```python
from build123d import *

# Parameters (mm, degrees)
BOSS_EXTRUDE1_DEPTH = 2
SKETCH2_R           = 2
CUT_EXTRUDE1_DEPTH  = 3
SKETCH6_W           = 5
SKETCH6_H           = 30
BOSS_EXTRUDE2_DEPTH = 10
FILLET1_R           = 5
FILLET2_R           = 3


with BuildPart() as part:
    # Sketch1 → Boss-Extrude1 (new body)
    with BuildSketch(Plane.XY):
        with BuildLine():
            Line((-43, 260), (43, 260))
            ThreePointArc((43, 260), (50.071067812, 262.928932188), (53, 270))
            Line((53, 270), (53, 350))
            ThreePointArc((53, 350), (50.071067812, 357.071067812), (43, 360))
            Line((43, 360), (-43, 360))
            ThreePointArc((-43, 360), (-50.071067812, 357.071067812), (-53, 350))
            Line((-53, 350), (-53, 270))
            ThreePointArc((-53, 270), (-50.071067812, 262.928932188), (-43, 260))
        make_face()
    extrude(amount=-BOSS_EXTRUDE1_DEPTH)

    # Sketch2 → Cut-Extrude1 (cut)
    with BuildSketch(Plane(origin=(0, 0, -2), x_dir=(-1, 0, 0), z_dir=(0, 0, -1))):
        with Locations((46, 267)):
            Circle(SKETCH2_R)
        with Locations((-46, 267)):
            Circle(SKETCH2_R)
        with Locations(Location((-46, 353, 0), (0, 0, 180))):
            Circle(SKETCH2_R)
        with Locations(Location((46, 353, 0), (0, 0, 180))):
            Circle(SKETCH2_R)
    extrude(amount=-CUT_EXTRUDE1_DEPTH, mode=Mode.SUBTRACT)

    # Sketch6 → Boss-Extrude2 (add)
    with BuildSketch(Plane.XY):
        with Locations((0, 310)):
            Rectangle(SKETCH6_W, SKETCH6_H)
    extrude(amount=BOSS_EXTRUDE2_DEPTH)

    # Fillet1
    fillet1_edges = [part.edges().sort_by_distance(p)[0] for p in [
        (0, 295, 10),
        (0, 325, 10),
    ]]
    fillet(fillet1_edges, radius=FILLET1_R)

    # Fillet2
    fillet2_edges = [part.edges().sort_by_distance(p)[0] for p in [
        (0, 295, 0),
        (0, 325, 0),
    ]]
    fillet(fillet2_edges, radius=FILLET2_R)


solid = part.part
```
For this review, take the finished solid that the model builds, in its own axes (mm). A direction names the side the tool comes from. Round coordinates to 2 decimals unless told otherwise and drop trailing zeros. Write each loop counter-clockwise with the first axis right and the second up, starting at its lowest first coordinate (ties: lowest second). Pieces come first, ordered by that corner, then holes. Notation, with made-up numbers: M 68.5,14 L 84.5,14 A21 cw 84.5,42 Z; hole C 3.5,30.25 d7. An arc over 180 degrees is marked long. One line per item, written item: value. Start each with the question number.
(1) Insertion check: pin 1 (3 mm diameter, centred on y = 283.5, z = 0.5, fed in from +X); pin 2 (5 mm diameter, centred on x = 46, y = 267, fed in from +Z); pin 3 (0.6 mm diameter, centred on x = -1, z = 4, fed in from -Y); pin 4 (0.6 mm diameter, centred on x = 1, z = 4, fed in from +Y). Each pin has a flat end and moves straight along its axis. Give the tip position at first contact, or say it passes through.
(2) We need section D-D (z = 8.75). Give the boundary of the cut face in (x, y), and give its area (3 significant figures).
(3) Machinability: for faces 1 (the flat face through (2.5, 310, 5)), 2 (the cylindrical face through (-49.99, 357.15, -0.99)), which of the approach directions +Z, -Z, +X, -X, +Y, -Y give a long, thin tool a straight path to every point of the face, cutting with its end or side? Answer none if there is none.
(4) We need section C-C (x = -35). Give the boundary of the cut face in (y, z), and give its area (3 significant figures).
(5) The part is to be moulded in two halves that separate along Y. For faces 3 (the flat face through (-2.5, 310, 5)), 4 (the cylindrical face through (46, 265, -1)), 5 (the cylindrical face through (-50.15, 263.01, -0.99)), say which applies: released by +Y, released by -Y, zero draft, split by the parting line, or undercut.
(6) We need section B-B (x = -46). Give the boundary of the cut face in (y, z).
(7) Wall thickness on line 1 (X direction, y = 353, z = -0.85); line 2 (Y direction, x = 46, z = -0.4); line 3 (X direction, y = 320.5, z = 4.5): over which ranges is each line inside the solid? List them lowest first.
(8) We need section A-A (y = 353). Give the boundary of the cut face in (x, z), and give its area (3 significant figures).
Result:
1. pin 1: x = 53
1. pin 2: z = 0
1. pin 3: y = 295
1. pin 4: y = 325
2. outline: M -2.5,296.69 L 2.5,296.69 L 2.5,323.31 L -2.5,323.31 Z
2. area: 133 mm²
3. face 1: +Z, +X, +Y, -Y
3. face 2: +Z, -Z, -X, +Y
4. outline: M 260,-2 L 360,-2 L 360,0 L 260,0 Z
4. area: 200 mm²
5. face 3: zero draft
5. face 4: undercut
5. face 5: released by -Y
6. outline: M 260.46,-2 L 265,-2 L 265,0 L 260.46,0 Z; M 269,-2 L 351,-2 L 351,0 L 269,0 Z; M 355,-2 L 359.54,-2 L 359.54,0 L 355,0 Z
7. line 1: -52.54 to -48, -44 to 44, 48 to 52.54
7. line 2: 260.46 to 265, 269 to 351, 355 to 359.54
7. line 3: -2.5 to 2.5
8. outline: M -52.54,-2 L -48,-2 L -48,0 L -52.54,0 Z; M -44,-2 L 44,-2 L 44,0 L -44,0 Z; M 48,-2 L 52.54,-2 L 52.54,0 L 48,0 Z
8. area: 194 mm²
